Here's how the part is built. I have some questions about the finished solid (model axes, mm). A direction names the side the tool comes from. Give positions to 0.01 mm unless a question says otherwise; leave off trailing zeros. Order: outer loops, then holes, each group sorted by start corner. A loop starts at its lowest first (then second) coordinate and runs counter-clockwise, first axis right, second up.
from build123d import *

# Parameters (mm, degrees)
BOSS_EXTRUDE1_DEPTH = 1.65
BOSS_EXTRUDE2_START = 2.95
SKETCH2_R           = 3.575
BOSS_EXTRUDE2_DEPTH = 2.95
SKETCH3_R           = 2.3
CUT_EXTRUDE1_DEPTH  = 2.95
SKETCH4_R           = 0.475
CUT_EXTRUDE2_DEPTH  = 1.65


with BuildPart() as part:
    # Sketch1 → Boss-Extrude1 (new body)
    with BuildSketch(Plane.XY):
        with BuildLine():
            Line((-15.178752219, 1.9), (0, 3.575))
            ThreePointArc((0, 3.575), (3.575, 0), (0, -3.575))
            Line((0, -3.575), (-15.178752219, -1.9))
            ThreePointArc((-15.178752219, -1.9), (-17.078752219, 0), (-15.178752219, 1.9))
        make_face()
    extrude(amount=BOSS_EXTRUDE1_DEPTH)

    # Sketch2 → Boss-Extrude2 (add)
    with BuildSketch(Plane(origin=(0, 0, 0), x_dir=(-1, 0, 0), z_dir=(0, 0, -1)).offset(BOSS_EXTRUDE2_START)):
        Circle(SKETCH2_R)
    extrude(amount=-BOSS_EXTRUDE2_DEPTH)

    # Sketch3 → Cut-Extrude1 (cut)
    with BuildSketch(Plane(origin=(0, 0, -2.95), x_dir=(-1, 0, 0), z_dir=(0, 0, -1))):
        Circle(SKETCH3_R)
    extrude(amount=-CUT_EXTRUDE1_DEPTH, mode=Mode.SUBTRACT)

    # Sketch4 → Cut-Extrude2 (cut)
    with BuildSketch(Plane.XY.offset(1.65)):
        with Locations((-13.103752219, 0)):
            Circle(SKETCH4_R)
    extrude(amount=-CUT_EXTRUDE2_DEPTH, mode=Mode.SUBTRACT)


solid = part.part
Q1. I need wall thicknesses on L1, parallel to Y at x = 0, z = -1.6 (3 decimals); L2, parallel to Z at x = -14.5, y = 0.25; L3, parallel to X at y = -1.75, z = -1.2. Which ranges of each line are inside material? Lowest first, please.
Filled sheet:
L1: y = -3.575 to -2.3, 2.3 to 3.575
L2: z = 0 to 1.65
L3: x = -3.12 to -1.49, 1.49 to 3.12
Q2. I'm going to push flat-ended pins straight in: P1, Ø1.4, axis at x = 0.5, y = 0.5, coming from the -Z side; P2, Ø2, axis at x = -11, z = 0.5, coming from the +Y side. Where does each tip first touch, or does it pass through?
Filled sheet:
P1: stops at z = 0
P2: stops at y = 2.47
Q3. Thinking about a two-plate mould opening in Y: for faces 1 (the face through (-9, 0, 0)), 2 (the face through (-17.08, -0.04, 0.81)), 3 (the face through (1.825, -1.4, -1.496)), 4 (the face through (0, 0, 0)), which applies, released by +Y, released by -Y, zero draft, split by the parting line, or undercut?
Filled sheet:
face 1: zero draft
face 2: split by the parting line
face 3: undercut
face 4: undercut
Q4. For faces 5 (the face through (-7, 0, 1.65)), 6 (the face through (3.57, 0.16, -1.19)), which set-ups out of +Z, -Z, +X, -X, +Y, -Y let a thin tool reach every point of the face, with its end or its side?
Filled sheet:
face 5: +Z, +X, -X, +Y, -Y
face 6: -Z
Q5. If we section it at B-B on z = -1.5: List the corners of the cut face in (x, y) for me (3 decimals), plus the area to 3 significant figures.
Filled sheet:
outline: circle Ø7.15 at (0, 0); hole circle Ø4.6 at (0, 0)
area: 23.5 mm2
Q6. If we section it at C-C on x = 1.75: List the corners of the cut face in (y, z) for me, plus the area to 3 significant figures.
Filled sheet:
outline: (-3.12, -2.95) - (-1.49, -2.95) - (-1.49, 0) - (1.49, 0) - (1.49, -2.95) - (3.12, -2.95) - (3.12, 1.65) - (-3.12, 1.65) - close
area: 19.9 mm2
Q7. If we section it at A-A on y = 0: List the corners of the cut face in (x, z) for me (3 decimals).
Filled sheet:
outline: (-17.079, 0) - (-13.579, 0) - (-13.579, 1.65) - (-17.079, 1.65) - close; (-12.629, 0) - (-3.575, 0) - (-3.575, -2.95) - (-2.3, -2.95) - (-2.3, 0) - (2.3, 0) - (2.3, -2.95) - (3.575, -2.95) - (3.575, 1.65) - (-12.629, 1.65) - close
Q8. If we section it at D-D on y = 2.5: List the corners of the cut face in (x, z) for me.
Filled sheet:
outline: (-9.74, 0) - (-2.56, 0) - (-2.56, -2.95) - (2.56, -2.95) - (2.56, 1.65) - (-9.74, 1.65) - close
